Here's how the part is built. I have some questions about the finished solid (model axes, mm). Face numbers are marked on the shaded views. A direction names the side the tool comes from. Round coordinates to 2 decimals unless told otherwise and drop trailing zeros. Order: outer loops, then holes, each group sorted by start corner. A loop starts at its lowest first (then second) coordinate and runs counter-clockwise, first axis right, second up. Notation, with made-up numbers: (39, 34) - (73, 34) arc R12 ccw to (73, 45) - close; hole circle Ø3 at (39, -33.75). An arc over 180 degrees is marked (long way). Answer as a JSON object with one key per item and string values.
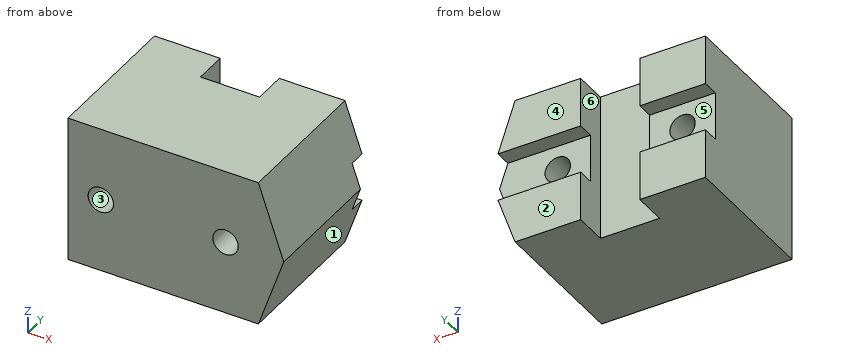
```python
from build123d import *

# Parameters (mm, degrees)
ESTRUSIONE_ESTRUSIONE1_DEPTH = 114
TAGLIO_ESTRUSIONE3_DEPTH     = 13
SCHIZZO6_W                   = 46.601982298
SCHIZZO6_H                   = 116
TAGLIO_ESTRUSIONE4_DEPTH     = 26
SCHIZZO7_R                   = 10
TAGLIO_ESTRUSIONE5_DEPTH     = 159.263069137


with BuildPart() as part:
    # Schizzo1 → Estrusione-Estrusione1 (new body)
    with BuildSketch(Plane(origin=(0, 0, 0), x_dir=(1, 0, 0), z_dir=(0, 1, 0))):
        Polygon((-107.155023459, -58), (-107.155023459, 58), (42.844976541, 58), (62.844976541, 0), (42.844976541, -58), align=None)
    extrude(amount=ESTRUSIONE_ESTRUSIONE1_DEPTH)

    # Schizzo3 → Taglio-Estrusione3 (cut)
    with BuildSketch(Plane(origin=(0, 114, 0), x_dir=(1, 0, 0), z_dir=(0, 1, 0))):
        Polygon((-107.155023459, -19), (-107.155023459, 19), (56.293252403, 19), (62.844976541, 0), (56.293252403, -19), align=None)
    extrude(amount=-TAGLIO_ESTRUSIONE3_DEPTH, mode=Mode.SUBTRACT)

    # Schizzo6 → Taglio-Estrusione4 (cut)
    with BuildSketch(Plane(origin=(0, 114, 0), x_dir=(1, 0, 0), z_dir=(0, 1, 0))):
        with Locations((-32.155023459, 0)):
            Rectangle(SCHIZZO6_W, SCHIZZO6_H)
    extrude(amount=-TAGLIO_ESTRUSIONE4_DEPTH, mode=Mode.SUBTRACT)

    # Schizzo7 → Taglio-Estrusione5 (cut, through all)
    with BuildSketch(Plane(origin=(0, 101, 0), x_dir=(1, 0, 0), z_dir=(0, 1, 0))):
        with Locations(Location((-81.305519034, 0, 0), (0, 0, 270))):
            Circle(SCHIZZO7_R)
        with Locations(Location((16.995472115, 0, 0), (0, 0, 90))):
            Circle(SCHIZZO7_R)
    extrude(amount=-TAGLIO_ESTRUSIONE5_DEPTH, mode=Mode.SUBTRACT)


solid = part.part
```
1. Thinking about a two-plate mould opening in Z: for the marked faces 1, 2 and 3, which applies, pulls with the +Z half, pulls with the -Z half, needs draft (parallel to the pull), parting line crosses it, or undercut?
Responses:
{"face 1": "pulls with the -Z half", "face 2": "needs draft", "face 3": "undercut"}
2. Imagine slicing it at D-D (z = 42). List the corners of the cut face in (x, y) for me, plus the area to 3 significant figures.
Responses:
{"outline": "(-107.16, 0) - (48.36, 0) - (48.36, 114) - (-8.85, 114) - (-8.85, 88) - (-55.46, 88) - (-55.46, 114) - (-107.16, 114) - close", "area": "16,500 mm2"}
3. If I drill on L1, parallel to X at y = 49, z = 0; L2, parallel to X at y = 41, z = -8; L3, parallel to Y at x = -13, z = 27.5, over which ranges is the centre line in solid material (lowest first)? Write a range as [from, to].
Responses:
{"L1": "[-107.16, -91.31], [-71.31, 7], [27, 62.84]", "L2": "[-107.16, -87.31], [-75.31, 11], [23, 60.09]", "L3": "[0, 88]"}
4. Imagine slicing it at B-B (x = -63). List the corners of the cut face in (y, z) for me.
Responses:
{"outline": "(0, -58) - (114, -58) - (114, -19) - (101, -19) - (101, 19) - (114, 19) - (114, 58) - (0, 58) - close"}
5. Imagine slicing it at C-C (y = 65.5). List the corners of the cut face in (x, z) for me.
Responses:
{"outline": "(-107.16, -58) - (42.84, -58) - (62.84, 0) - (42.84, 58) - (-107.16, 58) - close; hole circle Ø20 at (-81.31, 0); hole circle Ø20 at (17, 0)"}
6. Imagine slicing it at A-A (z = -3). List the corners of the cut face in (x, y) for me.
Responses:
{"outline": "(-107.16, 0) - (-90.84, 0) - (-90.84, 101) - (-107.16, 101) - close; (-71.77, 0) - (7.46, 0) - (7.46, 101) - (-8.85, 101) - (-8.85, 88) - (-55.46, 88) - (-55.46, 101) - (-71.77, 101) - close; (26.53, 0) - (61.81, 0) - (61.81, 101) - (26.53, 101) - close"}
7. For P1, Ø14, axis at x = -41.5, z = 21.5, coming from the +Y side; P2, Ø21, axis at y = 102, z = 24.5, coming from the +X side; P3, Ø18, axis at x = -81.31, z = 0, coming from the +Y side; P4, Ø10, axis at y = 28.5, z = -18, coming from the +X side, each with a flat end and sliding along its axis, tell me the tip position at first contact or that it passes through.
Responses:
{"P1": "y = 88", "P2": "x = 58", "P3": "through", "P4": "x = 58.36"}
8. For the marked faces 4, 5 and 6, which set-ups out of +Z, -Z, +X, -X, +Y, -Y let a thin tool reach every point of the face, with its end or its side?
Responses:
{"face 4": "+Z, -Z, +X, -X, +Y", "face 5": "+X, -X, +Y", "face 6": "+Z, -Z, +Y"}
